from build123d import *

# Parameters (mm, degrees)
F0_W     = 152.4
F0_H     = 50.8
F1_DEPTH = 152.4
F2_T     = -1.524


with BuildPart() as f1:
    # F0 (on Front) → F1 (new body, symmetric)
    with BuildSketch(Plane.XZ):
        with Locations((-36.709375, 8.207178)):
            Rectangle(F0_W, F0_H)
    extrude(amount=F1_DEPTH, both=True)

    # F2
    f2_openings = [f1.faces().sort_by_distance(p)[0] for p in [
        (-36.709375, 0, 33.607178),
    ]]
    offset(amount=F2_T, openings=f2_openings)


solid = f1.part
Build history of the part. All positions in model axes, mm. A direction names the side the tool comes from. Round coordinates to 2 decimals unless told otherwise and drop trailing zeros. Write each loop counter-clockwise with the first axis right and the second up, starting at its lowest first coordinate (ties: lowest second). Pieces come first, ordered by that corner, then holes. Notation, with made-up numbers: M 23.25,-15.75 L 71.25,-15.75 A22 ccw 71.25,-1.75 Z; hole C 73,48 d10. An arc over 180 degrees is marked long. Answer in a Markdown table with one row per item.
1. Flat gauge pin, fed straight in: P1, Ø2, axis at x = -57, y = 15.5, coming from the +Z side. Where does the tip first touch, or does it go through?
Geometry check:
| item | result |
|---|---|
| P1 | z = -15.67 |
2. Saw through at A-A (z = 16.5). List the corners of the cut face in (x, y), and give its area (3 significant figures).
Geometry check:
| item | result |
|---|---|
| outline | M -112.91,-152.4 L 39.49,-152.4 L 39.49,152.4 L -112.91,152.4 Z; hole M -111.39,-150.88 L 37.97,-150.88 L 37.97,150.88 L -111.39,150.88 Z |
| area | 1,380 mm2 |
3. Which spindle directions (+Z, -Z, +X, -X, +Y, -Y) get a long thin tool onto all of the face, cutting with end or side? Do faces 4 (the face through (-111.385, -2, 9)), 5 (the face through (-38, -152.4, 9)). Say none if no direction does.
Geometry check:
| item | result |
|---|---|
| face 4 | +Z |
| face 5 | +Z, -Z, +X, -X, -Y |
4. Mould opens along Y. For faces 1 (the face through (-38, 150.876, 9)), 2 (the face through (-38, 152.4, 9)), 3 (the face through (-112.909, -2, 8)) say: +Y half, -Y half, draft (parallel to the pull), parting line (faces both ways), or undercut.
Geometry check:
| item | result |
|---|---|
| face 1 | undercut |
| face 2 | +Y half |
| face 3 | draft |
5. Saw through at B-B (x = -83.5). List the corners of the cut face in (y, z).
Geometry check:
| item | result |
|---|---|
| outline | M -152.4,-17.19 L 152.4,-17.19 L 152.4,33.61 L 150.88,33.61 L 150.88,-15.67 L -150.88,-15.67 L -150.88,33.61 L -152.4,33.61 Z |
6. Saw through at C-C (y = -102). List the corners of the cut face in (x, z).
Geometry check:
| item | result |
|---|---|
| outline | M -112.91,-17.19 L 39.49,-17.19 L 39.49,33.61 L 37.97,33.61 L 37.97,-15.67 L -111.39,-15.67 L -111.39,33.61 L -112.91,33.61 Z |
7. Probe L1, parallel to Y at x = -69.5, z = -8.5; L2, parallel to X at y = 70, z = 10.5; L3, parallel to Z at x = 27, y = 76.5. List the from-to ranges inside material, lowest first. Write a range as [from, to].
Geometry check:
| item | result |
|---|---|
| L1 | [-152.4, -150.88], [150.88, 152.4] |
| L2 | [-112.91, -111.39], [37.97, 39.49] |
| L3 | [-17.19, -15.67] |
